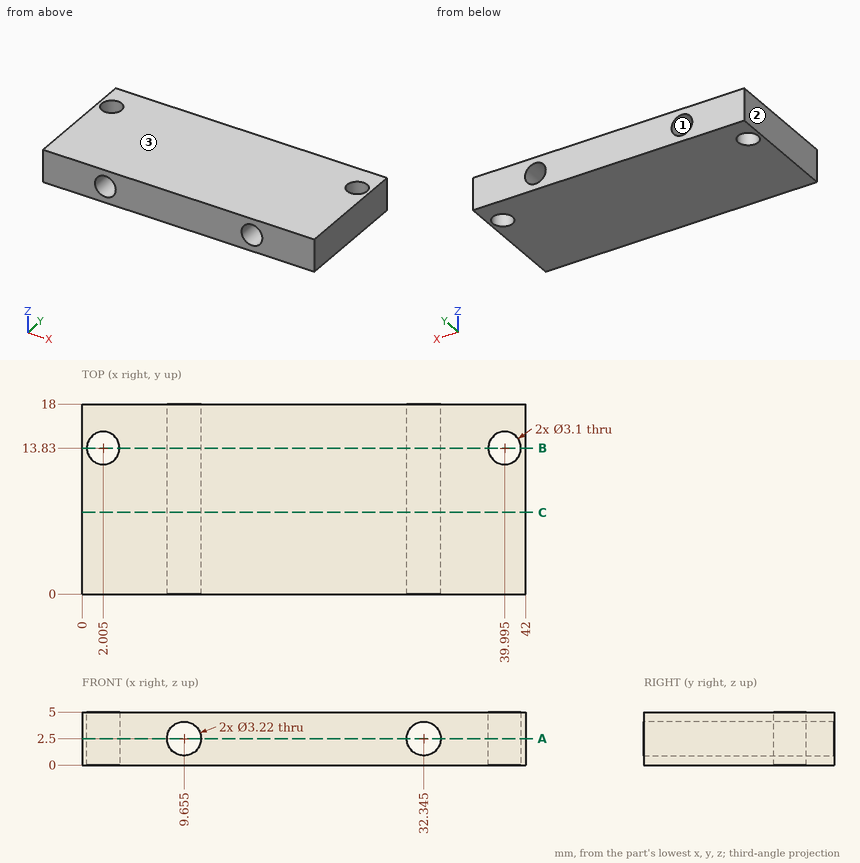
Verification items for this drawing (mm, ordinates from the low corner). Coordinates: 2 decimals unless noted, no trailing zeros. Loops run counter-clockwise (first coordinate to the right, second up) from the corner with the lowest first, then second, coordinate; pieces in that order, holes last. Notation, with made-up numbers: (15.5, 11.25) -> (24.5, 11.25) arc R19 ccw to (24.5, 23.25) -> close; hole circle Ø2 at (-39.5, -21.5). An arc over 180 degrees is marked (long way). Answer in a Markdown table with one row per item. Add a question column.
1. Section check A-A, the plane z = 2.5. Enter the section's corners in (x, y) (3 decimals), then the cut area to 3 significant figures.
2. Material ranges on probe 1 along X at (y, z) = (11.25, 2.6); probe 2 along Z at (x, y) = (32.5, 6); probe 3 along X at (y, z) = (4.5, 3.95), recorded low to high. Write a range as [from, to].
3. Depth check by flat-ended pin: P1, Ø3, axis at x = 2.005, y = 13.83, coming from the -Z side. Enter the tip coordinate at first touch or a pass-through.
4. Draft check along Z on the marked faces 1, 2 and 3. Enter one of: +Z half, -Z half, draft (parallel to the pull), parting line (faces both ways), or undercut.
5. Section check C-C, the plane y = 7.75. Enter the section's corners in (x, z) (3 decimals), then the cut area to 3 significant figures.
6. Section check B-B, the plane y = 13.83. Enter the section's corners in (x, z) (3 decimals).
Derived:
| question | item | result |
|---|---|---|
| 1 | outline | (0, 0) -> (8.045, 0) -> (8.045, 18) -> (0, 18) -> close; (11.265, 0) -> (30.735, 0) -> (30.735, 18) -> (11.265, 18) -> close; (33.955, 0) -> (42, 0) -> (42, 18) -> (33.955, 18) -> close; hole circle Ø3.1 at (2.005, 13.83); hole circle Ø3.1 at (39.995, 13.83) |
| 1 | area | 625 mm² |
| 2 | probe 1 | x = [0, 8.05], [11.26, 30.74], [33.95, 42] |
| 2 | probe 2 | z = [0, 0.9], [4.1, 5] |
| 2 | probe 3 | x = [0, 8.96], [10.35, 31.65], [33.04, 42] |
| 3 | P1 | passes through |
| 4 | face 1 | undercut |
| 4 | face 2 | draft |
| 4 | face 3 | +Z half |
| 5 | outline | (0, 0) -> (42, 0) -> (42, 5) -> (0, 5) -> close; hole circle Ø3.22 at (9.655, 2.5); hole circle Ø3.22 at (32.345, 2.5) |
| 5 | area | 194 mm² |
| 6 | outline | (0, 0) -> (0.455, 0) -> (0.455, 5) -> (0, 5) -> close; (3.555, 0) -> (38.445, 0) -> (38.445, 5) -> (3.555, 5) -> close; (41.545, 0) -> (42, 0) -> (42, 5) -> (41.545, 5) -> close; hole circle Ø3.22 at (9.655, 2.5); hole circle Ø3.22 at (32.345, 2.5) |
